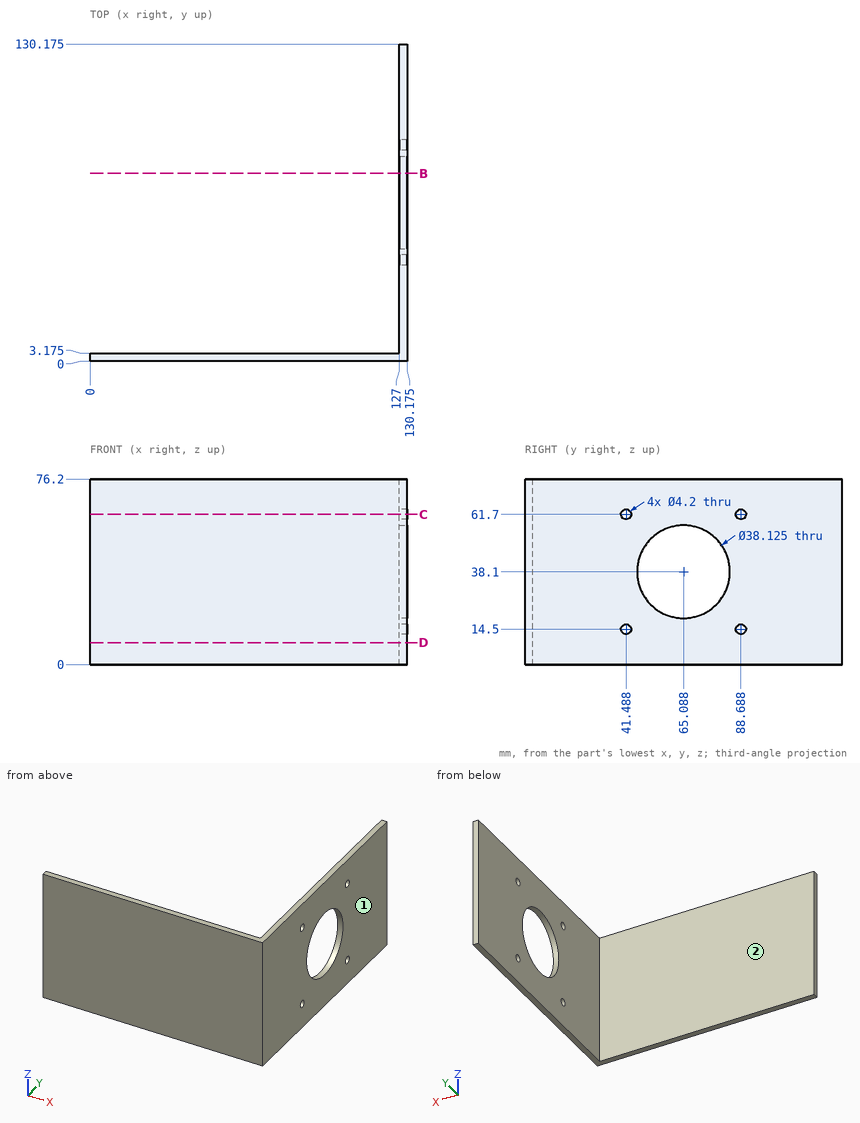
Input: dimensioned drawing with shaded views. Units: mm. Origin: part minimum x, y, z. A direction names the side the tool comes from. Give positions to 0.01 mm unless a question says otherwise; leave off trailing zeros. Write each loop counter-clockwise with the first axis right and the second up, starting at its lowest first coordinate (ties: lowest second). Pieces come first, ordered by that corner, then holes.
1. Section query B-B, the plane y = 77. Return loops of the section in (x, z) (1 decimal).
2. Pin query (flat end, axial travel): P1, Ø8, axis at y = 85, z = 23, coming from the -X side; P2, Ø4, axis at x = 55, z = 35.5, coming from the +Y side (1 decimal). Return the tip coordinate at first contact, or that it passes through.
3. Line query: probe 1 along Y at (x, z) = (127.8, 61.7) (1 decimal); probe 2 along Y at (x, z) = (128, 14) (1 decimal); probe 3 along X at (y, z) = (66.5, 7) (1 decimal). Output: solid intervals per line, ascending.
4. Section query D-D, the plane z = 9. Return loops of the section in (x, y) (1 decimal).
5. Reachability of the marked faces 1 and 2 from +Z, -Z, +X, -X, +Y, -Y: full face, straight path, thin tool, end or side. Return the list, or none.
6. Section query C-C, the plane z = 61.7. Return loops of the section in (x, y) (1 decimal).
Computed:
1. outline: (127, 0) - (130.2, 0) - (130.2, 23.2) - (127, 23.2) - close; (127, 53) - (130.2, 53) - (130.2, 76.2) - (127, 76.2) - close
2. P1: stops at x = 127
2. P2: stops at y = 3.2
3. probe 1: y = 0 to 39.4, 43.6 to 86.6, 90.8 to 130.2
3. probe 2: y = 0 to 39.4, 43.5 to 86.6, 90.7 to 130.2
3. probe 3: x = 127 to 130.2
4. outline: (0, 0) - (130.2, 0) - (130.2, 130.2) - (127, 130.2) - (127, 3.2) - (0, 3.2) - close
5. face 1: +Z, -Z, +X, +Y, -Y
5. face 2: +Z, -Z, -X, +Y
6. outline: (0, 0) - (130.2, 0) - (130.2, 39.4) - (127, 39.4) - (127, 3.2) - (0, 3.2) - close; (127, 43.6) - (130.2, 43.6) - (130.2, 86.6) - (127, 86.6) - close; (127, 90.8) - (130.2, 90.8) - (130.2, 130.2) - (127, 130.2) - close
